Part model, mm, in its own coordinate system. A direction names the side the tool comes from. Give positions to 0.01 mm unless a question says otherwise; leave off trailing zeros. Write each loop counter-clockwise with the first axis right and the second up, starting at its lowest first coordinate (ties: lowest second). Pieces come first, ordered by that corner, then holes. Notation, with made-up numbers: (-22, 87.5) - (16, 87.5) arc R13 cw to (16, 101.5) - close; hole circle Ø9 at (48.5, 77.5). An arc over 180 degrees is marked (long way). Answer as a JSON object with one key per item and string values. Group by question number.
Autodesk Inventor part; units mm, degrees
ref_plane "YZ Plane" through (0, 0, 0) normal (1, 0, 0) x (0, 1, 0)
ref_plane "XZ Plane" through (0, 0, 0) normal (0, 1, 0) x (-1, 0, 0)
ref_plane "XY Plane" through (0, 0, 0) normal (0, 0, 1) x (1, 0, 0)
sketch "Sketch1" plane through (0, 0, 0) normal (0, 0, 1) x (1, 0, 0)
  line L0 (-139.7, 31.75) -> (139.7, 31.75)
  line L1 (139.7, 31.75) -> (139.7, -31.75)
  line L2 (139.7, -31.75) -> (-139.7, -31.75)
  line L3 (-139.7, -31.75) -> (-139.7, 31.75)
  point P0 (0, 0)
  point P1 (0, 31.75)
  point P2 (139.7, 0)
  dimension "d0" = 279.4
  dimension "d1" = 63.5
extrude "Extrusion1" add sketch "Sketch1" along normal blind 43.18
sketch "Sketch2" plane through (0, 0, 43.18) normal (0, 0, 1) x (1, 0, 0)
  line L0 (-139.7, -31.75) -> (139.7, -31.75)
  line L1 (-138.1125, 30.1625) -> (138.1125, 30.1625)
  line L2 (138.1125, 30.1625) -> (138.1125, -31.75)
  line L3 (138.1125, -31.75) -> (-138.1125, -31.75)
  line L4 (-138.1125, -31.75) -> (-138.1125, 30.1625)
  line L5 (139.7, -31.75) -> (139.7, 31.75)
  line L6 (139.7, 31.75) -> (-139.7, 31.75)
  line L7 (-139.7, 31.75) -> (-139.7, -31.75)
  point P0 (0, 0)
  point P1 (-138.1125, -31.75)
  dimension "d4" = 1.5875
  dimension "d5" = 1.5875
  dimension "d6" = 1.5875
extrude "Extrusion2" cut sketch "Sketch2" against normal up to surface (43.18 mm away) contours L4 L1 L2 L0
sketch "Sketch3" plane through (-138.1125, -31.75, 43.18) normal (1, 0, 0) x (0, 0, -1)
  circle A0 centre (21.59, 41.5925) radius 5.05
  line L0 (0, 61.9125) -> (43.18, 61.9125)
  circle A1 centre (21.59, 21.2725) radius 1.5875
  line L1 (43.18, 63.5) -> (0, 63.5)
  point P0 (43.18, 31.75)
  point P1 (21.59, 63.5)
  dimension "d9" = 10.1
  dimension "d10" = 20.32
  dimension "d13" = 3.175
  dimension "d15" = 20.32
extrude "Extrusion3" cut sketch "Sketch3" along normal through all both and the other way through all
sketch "Sketch4" plane through (139.7, -31.75, 0) normal (1, 0, 0) x (0, 0, -1)
  circle A0 centre (-10.16, 26.3525) radius 2.3813
  line L0 (0, 63.5) -> (-43.18, 63.5) construction
  line L1 (-21.59, 63.5) -> (-21.59, -3.1611) construction
  line L2 (0, 0) -> (0, 63.5)
  circle A1 centre (-21.59, 41.5925) radius 5.05
  circle A2 centre (-33.02, 26.3525) radius 2.3813
  point P0 (0, 31.75)
  dimension "d16" = 10.16
  dimension "d17" = 15.24
  dimension "d18" = 4.7625
extrude "Extrusion4" cut sketch "Sketch4" against normal up to surface (1.5875 mm away) contours A0 | A2
sketch "Sketch5" plane through (-139.7, -31.75, 0) normal (-1, 0, 0) x (0, 0, 1)
  circle A0 centre (21.59, 41.5925) radius 5.05 construction
  line L0 (21.59, 41.5925) -> (21.59, 66.4825) construction
  line L1 (21.59, 41.5925) -> (51.2225, 41.5925) construction
  circle A1 centre (37.09, 57.0925) radius 1.5875
  circle A2 centre (6.09, 57.0925) radius 1.5875
  circle A3 centre (37.09, 26.0925) radius 1.5875
  circle A4 centre (6.09, 26.0925) radius 1.5875
  point P0 (0, 31.75)
  dimension "d21" = 3.175
  dimension "d22" = 15.5
  dimension "d23" = 15.5
extrude "Extrusion5" cut sketch "Sketch5" against normal up to surface (1.5875 mm away)
properties part number "Bracket"
1) Saw through at C-C (x = -66). List the corners of the cut face in (y, z).
2) Drill centre lines: line 1 along X through (y, z) = (-8.5, 12); line 2 along Y through (x, z) = (11.5, 25); line 3 along Y through (x, z) = (-139, 21). Where is each one in solid material? Low to high. Write a range as from..to.
3) Saw through at A-A (y = -26). List the corners of the cut face in (x, z).
4) Saw through at B-B (z = 33.02). List the corners of the cut face in (x, y).
5) Which spindle directions (+Z, -Z, +X, -X, +Y, -Y) get a long thin tool onto all of the face, cutting with end or side? Do faces 1 (the flat face through (-1, 31, 43.18)), 2 (the flat face through (-138.112, -1, 22)), 3 (the cylindrical face through (138.917, -3.788, 11.915)). Say none if no direction does.
6) Drop flat-ended pins along their axis: P1, Ø2.5, axis at y = 25.34, z = 37.09, coming from the -X side; P2, Ø21.5, axis at x = 12.5, z = 28.5, coming from the -Y side; P3, Ø3, axis at y = -5.4, z = 10.16, coming from the +X side. Give the stop position or say it passes through.
7) Two-plate mould, pull along Y, no slides. Class faces 4 (the flat face through (-2, 30.162, 22)), 5 (the cylindrical face through (138.895, 11.777, 16.925)), 6 (the flat face through (139.7, 0, 21)): +Y half, -Y half, draft (parallel to the pull), parting line (faces both ways), or undercut.
Checks:
{
 "1": {"outline": "(30.16, 0) - (31.75, 0) - (31.75, 43.18) - (30.16, 43.18) - close"},
 "2": {"line 1": "-139.7..-138.11, 138.11..139.7", "line 2": "30.16..31.75", "line 3": "-31.75..-11.95, -9..4.83, 14.86..31.75"},
 "3": {"outline": "(-139.7, 0) - (-138.11, 0) - (-138.11, 43.18) - (-139.7, 43.18) - close; (138.11, 0) - (139.7, 0) - (139.7, 43.18) - (138.11, 43.18) - close"},
 "4": {"outline": "(-139.7, -31.75) - (-138.11, -31.75) - (-138.11, 30.16) - (138.11, 30.16) - (138.11, -3.02) - (139.7, -3.02) - (139.7, 31.75) - (-139.7, 31.75) - close; (138.11, -31.75) - (139.7, -31.75) - (139.7, -7.78) - (138.11, -7.78) - close"},
 "5": {"face 1": "+Z, +X, -X, +Y, -Y", "face 2": "+Z, -Z, -Y", "face 3": "+X"},
 "6": {"P1": "x = 138.11", "P2": "y = 30.16", "P3": "x = -138.11"},
 "7": {"face 4": "-Y half", "face 5": "undercut", "face 6": "draft"}
}
